Geometry check sheet. Reference: the model listing, model coordinates, mm. Face numbers are marked on the shaded views. A direction names the side the tool comes from. Coordinates: 2 decimals unless noted, no trailing zeros. Order: outer loops, then holes, each group sorted by start corner. A loop starts at its lowest first (then second) coordinate and runs counter-clockwise, first axis right, second up. Notation, with made-up numbers: M -1,-21 L 29,-21 A25 ccw 29,4 Z; hole C 84.5,12 d2. An arc over 180 degrees is marked long. Use CSV: the item, a comma, the result in double quotes. Start each with the question number.
```python
from build123d import *

# Parameters (mm, degrees)
F0_R     = 19.05
F1_DEPTH = 38.1
F2_DEPTH = 25.4
F0_R_2   = 6.35
F3_DEPTH = 31.75


with BuildPart() as f1:
    # F0 (on Top) → F1 (new body)
    with BuildSketch(Plane.XY):
        with BuildLine():
            Line((-107.260471, 32.351975), (-112.290174, 32.854946))
            ThreePointArc((-112.290174, 32.854946), (-137.690174, 7.454946), (-112.290174, -17.945054))
            Line((-112.290174, -17.945054), (-107.260471, -17.442084))
            ThreePointArc((-107.260471, -17.442084), (-92.631658, -8.629294), (-86.890174, 7.454946))
            ThreePointArc((-86.890174, 7.454946), (-92.631658, 23.539186), (-107.260471, 32.351975))
        make_face()
        with Locations((-112.290174, 7.454946)):
            Circle(F0_R, mode=Mode.SUBTRACT)
    extrude(amount=F1_DEPTH)

    # F0 (on Top) → F2 (join)
    with BuildSketch(Plane.XY):
        with BuildLine():
            Line((14.709826, 20.154946), (-107.260471, 32.351975))
            ThreePointArc((-107.260471, 32.351975), (-92.631658, 23.539186), (-86.890174, 7.454946))
            ThreePointArc((-86.890174, 7.454946), (-92.631658, -8.629294), (-107.260471, -17.442084))
            Line((-107.260471, -17.442084), (14.709826, -5.245054))
            ThreePointArc((14.709826, -5.245054), (2.009826, 7.454946), (14.709826, 20.154946))
        make_face()
        with BuildLine():
            Line((-74.190174, 13.804946), (-23.390174, 13.804946))
            ThreePointArc((-23.390174, 13.804946), (-17.040174, 7.454946), (-23.390174, 1.104946))
            Line((-23.390174, 1.104946), (-74.190174, 1.104946))
            ThreePointArc((-74.190174, 1.104946), (-80.540174, 7.454946), (-74.190174, 13.804946))
        make_face(mode=Mode.SUBTRACT)
    extrude(amount=F2_DEPTH)

    # F0 (on Top) → F3 (join)
    with BuildSketch(Plane.XY):
        with BuildLine():
            ThreePointArc((27.409826, 7.454946), (23.690082, 16.435202), (14.709826, 20.154946))
            ThreePointArc((14.709826, 20.154946), (2.009826, 7.454946), (14.709826, -5.245054))
            ThreePointArc((14.709826, -5.245054), (23.690082, -1.52531), (27.409826, 7.454946))
        make_face()
        with Locations((14.709826, 7.454946)):
            Circle(F0_R_2, mode=Mode.SUBTRACT)
    extrude(amount=F3_DEPTH)


solid = f1.part
```
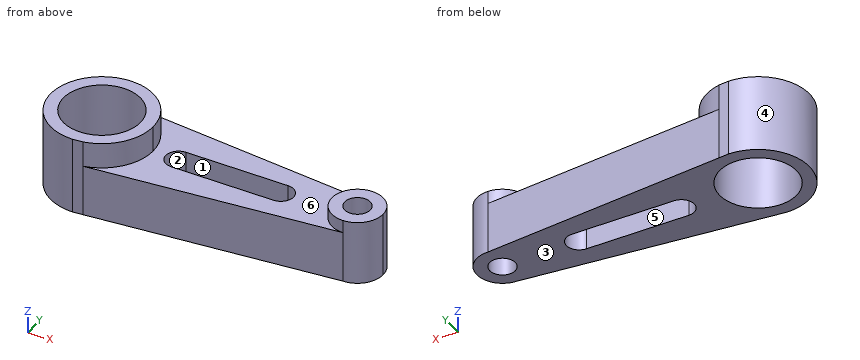
1) Section check B-B on x = -45.5. Record the boundary of the cut face in (y, z), then the cut area to 3 significant figures.
2) Gauge pin test, flat ends, axial feed: P1, Ø23, axis at x = -112.29, y = 7.45, coming from the +Z side; P2, Ø1, axis at x = -40.5, y = 15, coming from the +Z side; P3, Ø7.5, axis at x = 18, y = 1.5, coming from the +Z side; P4, Ø2, axis at y = 20, z = 25.5, coming from the -X side. Record the tip position at first contact, or that the pin passes through.
3) Set-up check for the marked faces 5 and 6: record each of +Z, -Z, +X, -X, +Y, -Y from which the full face is reachable in a straight line by a thin tool's end or side.
4) Material ranges on line 1 along X through (y, z) = (7.5, 25.5); line 2 along X through (y, z) = (7, 27); line 3 along Z through (x, y) = (-32.5, 1), recorded low to high.
5) Section check D-D on z = 34. Record the boundary of the cut face in (x, y), then the cut area to 3 significant figures.
6) Section check A-A on z = 18.5. Record the boundary of the cut face in (x, y), then the cut area to 3 significant figures.
7) Section check C-C on y = 3.5. Record the boundary of the cut face in (x, z), then the cut area to 3 significant figures.
8) Draft check along Y on the marked faces 1, 2, 3 and 4. Enter one of: +Y half, -Y half, draft (parallel to the pull), parting line (faces both ways), or undercut.
Results are:
1,outline,"M -11.27,0 L 1.1,0 L 1.1,25.4 L -11.27,25.4 Z; M 13.8,0 L 26.18,0 L 26.18,25.4 L 13.8,25.4 Z"
1,area,"628 mm²"
2,P1,"passes through"
2,P2,"stops at z = 25.4"
2,P3,"stops at z = 31.75"
2,P4,"stops at x = -134.91"
3,face 5,"+Z, -Z"
3,face 6,"+Z"
4,line 1,"x = -137.69 to -131.34, -93.24 to -86.89, 2.01 to 8.36, 21.06 to 27.41"
4,line 2,"x = -137.69 to -131.33, -93.25 to -86.89, 2.02 to 8.38, 21.04 to 27.4"
4,line 3,"z = 0 to 25.4"
5,outline,"M -112.29,-17.95 L -107.26,-17.44 A25.4 ccw -86.89,7.45 A25.4 ccw -107.26,32.35 L -112.29,32.85 A25.4 ccw Z; hole C -112.29,7.45 d38.1"
5,area,"886 mm²"
6,outline,"M -112.29,-17.95 L 14.71,-5.25 A12.7 ccw 14.71,20.15 L -107.26,32.35 L -112.29,32.85 A25.4 ccw Z; hole C -112.29,7.45 d38.1; hole M -74.19,1.1 L -23.39,1.1 A6.35 ccw -23.39,13.8 L -74.19,13.8 A6.35 ccw Z; hole C 14.71,7.45 d12.7"
6,area,"4,070 mm²"
7,outline,"M -137.38,0 L -130.93,0 L -130.93,38.1 L -137.38,38.1 Z; M -93.66,0 L -79.16,0 L -79.16,25.4 L -87.2,25.4 L -87.2,38.1 L -93.66,38.1 Z; M -18.42,0 L 9.74,0 L 9.74,31.75 L 2.64,31.75 L 2.64,25.4 L -18.42,25.4 Z; M 19.68,0 L 26.78,0 L 26.78,31.75 L 19.68,31.75 Z"
7,area,"1,680 mm²"
8,face 1,"undercut"
8,face 2,"undercut"
8,face 3,"draft"
8,face 4,"parting line"
